The model under review builds one solid part; all positions refer to its coordinate system, in mm. A direction names the side the tool comes from. Round coordinates to 2 decimals unless told otherwise and drop trailing zeros. Loops run counter-clockwise (first coordinate to the right, second up) from the corner with the lowest first, then second, coordinate; pieces in that order, holes last. Notation, with made-up numbers: M 70,2 L 85,2 A34 ccw 85,36 Z; hole C 81,25 d9. An arc over 180 degrees is marked long. Return JSON: item names as keys, results as strings. Group by question number.
Q1. Consider section B-B (x = 18). State the section outline as (y, z) points, and give its area (3 significant figures).
Q2. Consider section D-D (y = -9). State the section outline as (x, z) points (3 decimals).
Q3. Clearance check with flat-ended pins moving along their axes: pin 1 Ø3 at (x, y) = (-13.5, 8) entering from -Z; pin 2 Ø7 at (y, z) = (12.5, 0) entering from -X; pin 3 Ø4 at (x, y) = (10, -26) entering from -Z; pin 4 Ø4 at (y, z) = (-6.5, 8.5) entering from -X. State where each tip first meets the part, or that it passes through.
Q4. Consider section C-C (z = -18). State the section outline as (x, y) points.
Q5. Consider section A-A (x = 0). State the section outline as (y, z) points (3 decimals), and give its area (3 significant figures).
Q6. Draft analysis for pull direction X (two halves, no side actions). For faces 1 (the face through (-1.968, 11, 0)), 2 (the face through (-0.43, 3.131, 16.063)), 3 (the face through (0, 10.7, 4.7)), state which applies: pulls with the +X half, pulls with the -X half, needs draft (parallel to the pull), parting line crosses it, or undercut.
Q7. For faces 4 (the face through (0, 0, 15)), 5 (the face through (0, 10.7, -4.7)), 6 (the face through (1.968, 11, 0)), list the 3-axis set-ups (+Z, -Z, +X, -X, +Y, -Y) from which the entire face can be reached by the end or side of a thin tool; tool diameter is ignored.
Q8. To check wall thickness, follow line 1 along Z through (x, y) = (0, 2); line 2 along Y through (x, z) = (3.5, -21). State the ranges of each line that lie inside material, in increasing order.
from build123d import *

# Parameters (mm, degrees)
SKETCH1_R                           = 22.86
BOSS_EXTRUDE1_DEPTH                 = 6.35
BOSS_EXTRUDE2_DEPTH                 = 8.89
SKETCH3_R                           = 10.795
BOSS_EXTRUDE3_DEPTH                 = 50.8
CHAMFER1_SIZE                       = 3.81
F_5_32_0_15625_DIAMETER_HOLE1_D     = 3.96875
F_5_32_0_15625_DIAMETER_HOLE1_DEPTH = 6.351
CIRPATTERN1_COUNT                   = 4


with BuildPart() as part:
    # Sketch1 → Boss-Extrude1 (new body)
    with BuildSketch(Plane(origin=(0, 0, 0), x_dir=(1, 0, 0), z_dir=(0, 1, 0))):
        Circle(SKETCH1_R)
    extrude(amount=BOSS_EXTRUDE1_DEPTH)

    # Sketch2 → Boss-Extrude2 (add)
    with BuildSketch(Plane(origin=(0, 6.35, 0), x_dir=(1, 0, 0), z_dir=(0, 1, 0))):
        with BuildLine():
            Line((1.9685, -4.266803107), (1.9685, 4.266803107))
            ThreePointArc((1.9685, 4.266803107), (0, 4.699), (-1.9685, 4.266803107))
            Line((-1.9685, 4.266803107), (-1.9685, -4.266803107))
            ThreePointArc((-1.9685, -4.266803107), (0, -4.699), (1.9685, -4.266803107))
        make_face()
    extrude(amount=BOSS_EXTRUDE2_DEPTH)

    # Sketch3 → Boss-Extrude3 (add)
    with BuildSketch(Plane.XZ):
        Circle(SKETCH3_R)
    extrude(amount=BOSS_EXTRUDE3_DEPTH)

    # Chamfer1
    chamfer1_edges = [part.edges().sort_by_distance(p)[0] for p in [
        (-10.795, 0, 0),
    ]]
    chamfer(chamfer1_edges, length=CHAMFER1_SIZE)

    # 5/32 (0.15625) Diameter Hole1
    with Locations(Plane(origin=(0, 6.35, 0), x_dir=(1, 0, 0), z_dir=(0, 1, 0))):
        with Locations((0, 18)):
            f_5_32_0_15625_diameter_hole1 = Hole(F_5_32_0_15625_DIAMETER_HOLE1_D / 2, depth=F_5_32_0_15625_DIAMETER_HOLE1_DEPTH)

    # CirPattern1: 5/32 (0.15625) Diameter Hole1 ×4 about axis
    cirpattern1_axis = Axis((0, 0, 0), (0, 1, 0))
    for i in range(1, CIRPATTERN1_COUNT):
        add(f_5_32_0_15625_diameter_hole1.rotate(cirpattern1_axis, i * 360 / CIRPATTERN1_COUNT), mode=Mode.SUBTRACT)


solid = part.part
Values:
{
 "1": {"outline": "M 0,-14.09 L 6.35,-14.09 L 6.35,-1.98 L 0,-1.98 Z; M 0,1.98 L 6.35,1.98 L 6.35,14.09 L 0,14.09 Z", "area": "154 mm2"},
 "2": {"outline": "C 0,0 d21.59"},
 "3": {"pin 1": "passes through", "pin 2": "stops at x = -1.97", "pin 3": "stops at z = -7.25", "pin 4": "stops at x = -8.62"},
 "4": {"outline": "M -14.09,0 L -1.98,0 L -1.98,6.35 L -14.09,6.35 Z; M 1.98,0 L 14.09,0 L 14.09,6.35 L 1.98,6.35 Z"},
 "5": {"outline": "M -50.8,-10.795 L -3.81,-10.795 L 0,-14.605 L 0,-16.016 L 6.35,-16.016 L 6.35,-4.699 L 15.24,-4.699 L 15.24,4.699 L 6.35,4.699 L 6.35,16.016 L 0,16.016 L 0,14.605 L -3.81,10.795 L -50.8,10.795 Z; M 0,-22.86 L 6.35,-22.86 L 6.35,-19.984 L 0,-19.984 Z; M 0,19.984 L 6.35,19.984 L 6.35,22.86 L 0,22.86 Z", "area": "1,430 mm2"},
 "6": {"face 1": "pulls with the -X half", "face 2": "undercut", "face 3": "parting line crosses it"},
 "7": {"face 4": "-Y", "face 5": "-Z, +Y", "face 6": "+Z, -Z, +X, +Y"},
 "8": {"line 1": "z = -22.86 to -19.98, -16.02 to 16.02, 19.98 to 22.86", "line 2": "y = 0 to 6.35"}
}
